Geometry: see drawing. Coordinates: mm, zero at the bounding-box minimum. Coordinates: 2 decimals unless noted, no trailing zeros. Order: outer loops, then holes, each group sorted by start corner. A loop starts at its lowest first (then second) coordinate and runs counter-clockwise, first axis right, second up. Notation, with made-up numbers: (-4.5, 42.25) -> (39.5, 42.25) arc R24 ccw to (39.5, 67.25) -> close; hole circle Ø4 at (-17.75, 43.5). An arc over 180 degrees is marked (long way). Use CSV: the item, a comma, the result in double quotes. Start each with the question number.
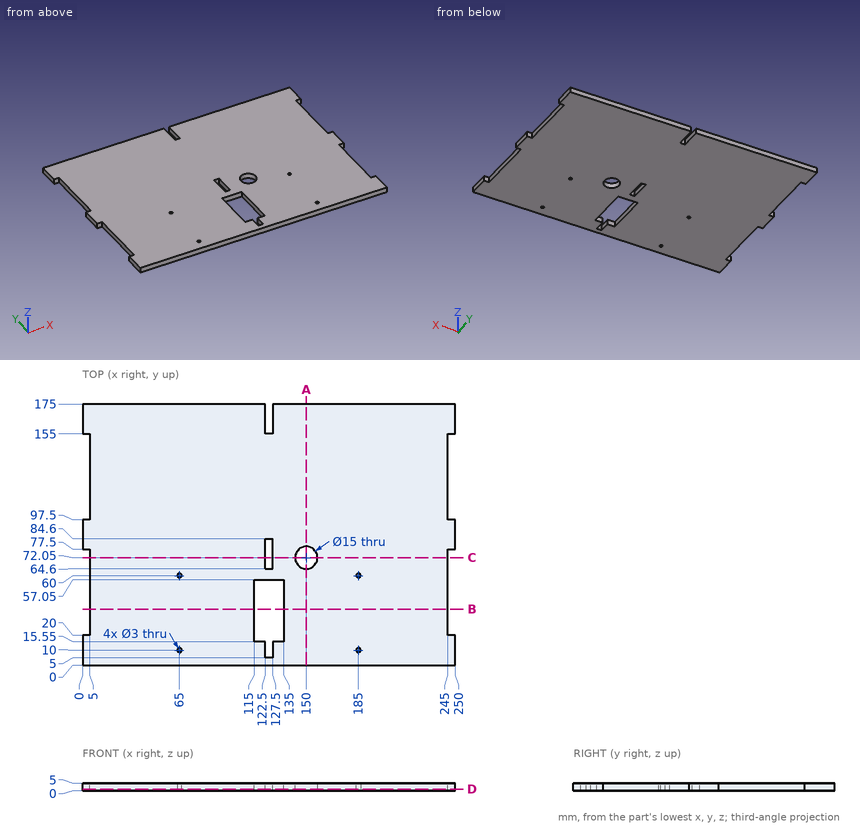
(1) Section B-B (y = 37.5). Return loops of the section in (x, z), then the cut area to 3 significant figures.
(2) Line query: line 1 (X direction, y = 60, z = 2.25); line 2 (Y direction, x = 126, z = 1.2); line 3 (Y direction, x = 150, z = 2.95). Output: solid intervals per line, ascending. Write a range as from..to.
(3) Section A-A (x = 150). Return loops of the section in (y, z), then the cut area to 3 significant figures.
(4) Section C-C (y = 72.05). Return loops of the section in (x, z), then the cut area to 3 significant figures.
(5) First-contact query: pin 1 (2 mm diameter, centred on y = 67.5, z = 1, fed in from +X); pin 2 (2.5 mm diameter, centred on y = 114, z = 3.5, fed in from -X). Flat tips, straight axial feed; report the tip coordinate or a pass-through.
(6) Section D-D (z = 0.9). State how many separate pieces and enclosed holes the cut face has, then the cut area to 3 significant figures.
Check sheet entries:
1,outline,"(5, 0) -> (115, 0) -> (115, 5) -> (5, 5) -> close; (135, 0) -> (245, 0) -> (245, 5) -> (135, 5) -> close"
1,area,"1,100 mm^2"
2,line 1,"x = 5..63.5, 66.5..183.5, 186.5..245"
2,line 2,"y = 0..5, 57.05..64.6, 84.6..155"
2,line 3,"y = 0..64.55, 79.55..175"
3,outline,"(0, 0) -> (64.55, 0) -> (64.55, 5) -> (0, 5) -> close; (79.55, 0) -> (175, 0) -> (175, 5) -> (79.55, 5) -> close"
3,area,"800 mm^2"
4,outline,"(5, 0) -> (122.5, 0) -> (122.5, 5) -> (5, 5) -> close; (127.5, 0) -> (142.5, 0) -> (142.5, 5) -> (127.5, 5) -> close; (157.5, 0) -> (245, 0) -> (245, 5) -> (157.5, 5) -> close"
4,area,"1,100 mm^2"
5,pin 1,"stops at x = 245"
5,pin 2,"stops at x = 5"
6,separate pieces,"1"
6,enclosed holes,"7"
6,area,"41,300 mm^2"
